from build123d import *

# Parameters (mm, degrees)
F0_W     = 57.15
F0_H     = 57.15
F1_DEPTH = 88.9
F2_W     = 23.8125
F2_H     = 23.8125
F3_DEPTH = 82.55
F4_W     = 23.8125
F4_H     = 23.8125
F5_DEPTH = 82.55
F6_W     = 23.8125
F6_H     = 23.8125
F7_DEPTH = 82.55
F8_W     = 23.8125
F8_H     = 23.8125
F9_DEPTH = 82.55


with BuildPart() as f1:
    # F0 (on Front) → F1 (new body)
    with BuildSketch(Plane.XZ):
        Rectangle(F0_W, F0_H)
    extrude(amount=F1_DEPTH)

    # F2 (on face) → F3 (cut)
    with BuildSketch(Plane.XZ.offset(88.9)):
        with Locations((-13.49375, 13.49375)):
            Rectangle(F2_W, F2_H)
    extrude(amount=-F3_DEPTH, mode=Mode.SUBTRACT)

    # F4 (on face) → F5 (cut)
    with BuildSketch(Plane.XZ.offset(88.9)):
        with Locations((13.49375, 13.49375)):
            Rectangle(F4_W, F4_H)
    extrude(amount=-F5_DEPTH, mode=Mode.SUBTRACT)

    # F6 (on face) → F7 (cut)
    with BuildSketch(Plane.XZ.offset(88.9)):
        with Locations((-13.49375, -13.49375)):
            Rectangle(F6_W, F6_H)
    extrude(amount=-F7_DEPTH, mode=Mode.SUBTRACT)

    # F8 (on face) → F9 (cut)
    with BuildSketch(Plane.XZ.offset(88.9)):
        with Locations((13.49375, -13.49375)):
            Rectangle(F8_W, F8_H)
    extrude(amount=-F9_DEPTH, mode=Mode.SUBTRACT)


solid = f1.part
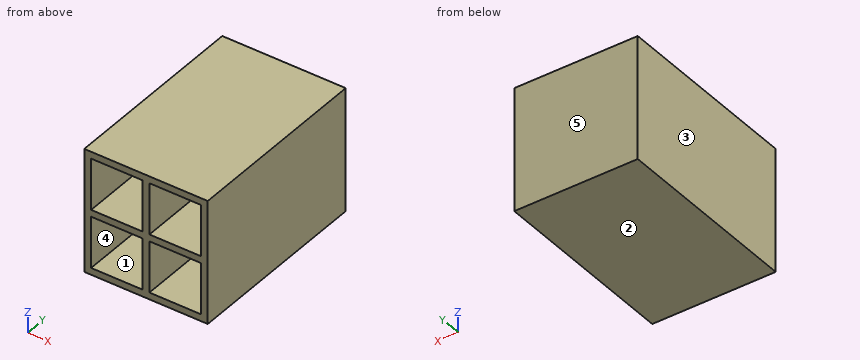
Verification items for the finished model (mm, model axes). Face numbers are marked on the shaded views. A direction names the side the tool comes from. Coordinates: 2 decimals unless noted, no trailing zeros. Write each loop counter-clockwise with the first axis right and the second up, starting at its lowest first coordinate (ties: lowest second). Pieces come first, ordered by that corner, then holes. Notation, with made-up numbers: (48, 45.5) -> (99, 45.5) arc R33 ccw to (99, 74.5) -> close; hole circle Ø10 at (83, 87). An arc over 180 degrees is marked (long way). One line per item, written item: value. Start each with the question number.
Q1. Thickness scan on L1, parallel to Z at x = 23, y = -12 (1 decimal); L2, parallel to Y at x = -9.5, z = 24. Record the ranges inside material, lowest first. Write a range as from..to.
Q2. Cross-section at A-A on y = -22. Enter the section's corners in (x, z) (1 decimal).
Q3. Access from +Z, -Z, +X, -X, +Y, -Y to the whole of each face (thin tool, end or side, straight path). Record for the marked faces 4 and 5.
Q4. Mould release check, pull along Z, two halves, no side actions. Record for the marked faces 1, 2 and 3: pulls with the +Z half, pulls with the -Z half, needs draft (parallel to the pull), parting line crosses it, or undercut.
Q5. Go/stop test with a flat-tipped pin: P1, Ø3, axis at x = -14, z = 16, coming from the -Y side. Record where the tip stops, or that it passes through.
Checked values:
1. L1: z = -28.6..-25.4, -1.6..1.6, 25.4..28.6
1. L2: y = -6.35..0
2. outline: (-28.6, -28.6) -> (28.6, -28.6) -> (28.6, 28.6) -> (-28.6, 28.6) -> close; hole (-25.4, -25.4) -> (-1.6, -25.4) -> (-1.6, -1.6) -> (-25.4, -1.6) -> close; hole (-25.4, 1.6) -> (-1.6, 1.6) -> (-1.6, 25.4) -> (-25.4, 25.4) -> close; hole (1.6, -25.4) -> (25.4, -25.4) -> (25.4, -1.6) -> (1.6, -1.6) -> close; hole (1.6, 1.6) -> (25.4, 1.6) -> (25.4, 25.4) -> (1.6, 25.4) -> close
3. face 4: -Y
3. face 5: +Z, -Z, +X, -X, +Y
4. face 1: undercut
4. face 2: pulls with the -Z half
4. face 3: needs draft
5. P1: stops at y = -6.35
